```python
from build123d import *

# Parameters (mm, degrees)
F1_DEPTH = 25.4


with BuildPart() as f1:
    # F0 (on Front) → F1 (new body)
    with BuildSketch(Plane.XZ):
        Polygon((-44.868574, -66.656321), (-34.102677, -38.775525), (32.936819, -39.698683), (45.380164, -66.460343), (67.723832, -66.460343), (22.177352, 49.990933), (0, 49.990933), (-22.180768, 49.990933), (-67.222965, -66.656321), align=None)
        Polygon((8.083392, 27.979204), (25.479969, -19.393079), (-26.656247, -19.393079), (-8.45656, 27.979204), align=None, mode=Mode.SUBTRACT)
    extrude(amount=F1_DEPTH)


solid = f1.part
```
Geometry: final body of the model. Coordinates: model frame, mm. A direction names the side the tool comes from. Coordinates: 2 decimals unless noted, no trailing zeros. Write each loop counter-clockwise with the first axis right and the second up, starting at its lowest first coordinate (ties: lowest second). Pieces come first, ordered by that corner, then holes. Notation, with made-up numbers: M 58,10.25 L 108,10.25 A30 ccw 108,35.25 Z; hole C 36.5,0 d9. An arc over 180 degrees is marked long. Use CSV: the item, a comma, the result in double quotes. Start each with the question number.
1. Cut plane B-B on y = -15. Return the cut outline in (x, z), plus the area to 3 significant figures.
2. Ray query, probe 1 along X at (y, z) = (-23.5, -50); probe 2 along Z at (x, y) = (2, -20); probe 3 along Z at (x, y) = (-2, -3.5). Return the intervals inside material, ascending.
3. Reachability of faces 4 (the face through (39.07, -12.52, -52.89)), 5 (the face through (-56, -13, -66.656)), 6 (the face through (16.66, -12.52, 4.62)) from +Z, -Z, +X, -X, +Y, -Y: full face, straight path, thin tool, end or side. Return the list, or none.
4. Mould query, pull axis X, two halves, no side actions, for faces 1 (the face through (56, -13, -66.46)), 2 (the face through (-17.684, -12.522, 3.961)), 3 (the face through (-44.39, -12.52, -7.52)). Classes: pulls with the +X half, pulls with the -X half, needs draft (parallel to the pull), parting line crosses it, or undercut.
5. First-contact query: P1, Ø12, axis at y = -9, z = -54, coming from the +X side; P2, Ø10, axis at x = -47.5, z = 5.5, coming from the -Y side; P3, Ø8, axis at y = -14, z = -11, coming from the -X side; P4, Ø11, axis at x = 56, y = -9.5, coming from the -Z side. Flat tips, straight axial feed; report the tip coordinate or a pass-through.
6. Cut plane A-A on z = 15.5. Return the cut outline in (x, y), plus the area to 3 significant figures.
7. Cut plane C-C on x = -12. Return the cut outline in (y, z).
Entries:
1,outline,"M -67.22,-66.66 L -44.87,-66.66 L -34.1,-38.78 L 32.94,-39.7 L 45.38,-66.46 L 67.72,-66.46 L 22.18,49.99 L -22.18,49.99 Z; hole M -26.66,-19.39 L 25.48,-19.39 L 8.08,27.98 L -8.46,27.98 Z"
1,area,"6,670 mm²"
2,probe 1,"-60.79 to -38.44, 37.73 to 61.29"
2,probe 2,"-39.27 to -19.39, 27.98 to 49.99"
2,probe 3,"-39.22 to -19.39, 27.98 to 49.99"
3,face 4,"-Z, +Y, -Y"
3,face 5,"-Z, +X, -X, +Y, -Y"
3,face 6,"+Y, -Y"
4,face 1,"needs draft"
4,face 2,"undercut"
4,face 3,"pulls with the -X half"
5,P1,"x = 65.2"
5,P2,"through"
5,P3,"x = -47.28"
5,P4,"z = -66.46"
6,outline,"M -35.5,-25.4 L -13.25,-25.4 L -13.25,0 L -35.5,0 Z; M 12.67,-25.4 L 35.67,-25.4 L 35.67,0 L 12.67,0 Z"
6,area,"1,150 mm²"
7,outline,"M -25.4,-39.08 L 0,-39.08 L 0,-19.39 L -25.4,-19.39 Z; M -25.4,18.76 L 0,18.76 L 0,49.99 L -25.4,49.99 Z"
